Source: CAD feature listing. Evaluate the final solid. Frame: model axes, mm. Face numbers are marked on the shaded views. A direction names the side the tool comes from. Coordinates: 2 decimals unless noted, no trailing zeros. Write each loop counter-clockwise with the first axis right and the second up, starting at its lowest first coordinate (ties: lowest second). Pieces come first, ordered by that corner, then holes. Notation, with made-up numbers: M -13,-39.5 L 41,-39.5 A28 ccw 41,-15.5 Z; hole C 4.25,24.5 d5. An arc over 180 degrees is marked long. One line per item, written item: value. Start each with the question number.
Item 1: Cut plane B-B, the plane y = -25. Output: boundary loops of the cut face in (x, z).
Item 2: Cut plane A-A, the plane x = 0. Output: boundary loops of the cut face in (y, z).
Item 3: Ray query, L1, parallel to Y at x = -4.5, z = -7.75; L2, parallel to Y at x = 6.5, z = -0.6; L3, parallel to Z at x = 29.5, y = -3. Return the intervals inside material, ascending. Write a range as from..to.
Item 4: Cut plane D-D, the plane x = -19. Output: boundary loops of the cut face in (y, z), then the cut area to 3 significant figures.
Item 5: Mould query, pull axis Y, two halves, no side actions, for the marked faces 1, 2, 3 and 4. Classes: released by +Y, released by -Y, zero draft, split by the parting line, or undercut.
Item 6: Pin query (flat end, axial travel): P1, Ø6.5, axis at x = -2, z = -14, coming from the +Y side; P2, Ø5.5, axis at x = -21.5, z = -22, coming from the -Y side; P3, Ø7, axis at x = 2.5, z = -8, coming from the +Y side; P4, Ø12, axis at x = 22.5, z = -6, coming from the +Y side. Return the tip coordinate at first contact, or that it passes through.
Item 7: Set-up query: the marked faces 5, 6 and 7. Return all of +Z, -Z, +X, -X, +Y, -Y with unobstructed straight access to the full face (end or side cutting, diameter ignored); none if empty.
Item 8: Cut plane C-C, the plane z = -6.75. Output: boundary loops of the cut face in (x, y), then the cut area to 3 significant figures.
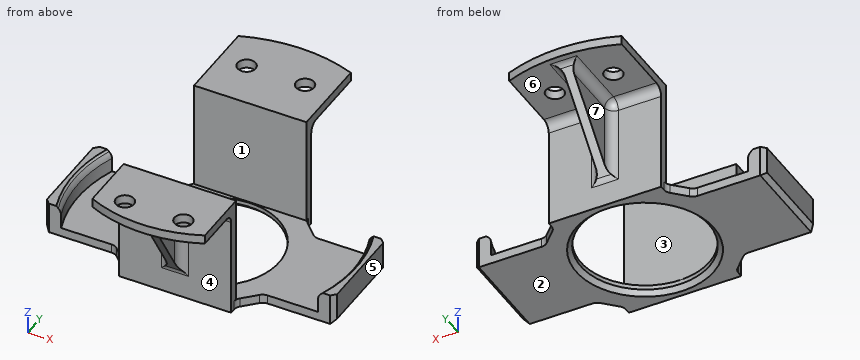
```python
from build123d import *

# Parameters (mm, degrees)
BOSS_EXTRUDE1_DEPTH     = 12.5
SKETCH2_R               = 45
SKETCH2_R_2             = 35
CUT_EXTRUDE_THIN1_DEPTH = 10
CUT_EXTRUDE1_DEPTH      = 10
BOSS_EXTRUDE2_DEPTH     = 32.275
SKETCH5_R               = 14.25
CUT_EXTRUDE2_DEPTH      = 40
CHAMFER1_SIZE           = 5
CHAMFER2_SIZE           = 1
BOSS_EXTRUDE3_DEPTH     = 5
CHAMFER3_SIZE           = 5
FILLET1_R               = 3
RIB2_REACH              = 56.318
SKETCH7_WALL_W          = 134.965083932
SKETCH7_WALL_H          = 2
RIB3_REACH              = 56.318
SKETCH8_WALL_W          = 131.736112932
SKETCH8_WALL_H          = 2
CUT_EXTRUDE3_DEPTH      = 55.318487934
CHAMFER4_SIZE           = 1
SKETCH10_R              = 2
CUT_EXTRUDE4_DEPTH      = 5
CHAMFER5_SIZE           = 1
FILLET2_R               = 2


with BuildPart() as part:
    # Sketch1 → Boss-Extrude1 (new, symmetric)
    with BuildSketch(Plane(origin=(0, 0, 0), x_dir=(0, 0, -1), z_dir=(1, 0, 0))):
        Polygon((0, 35), (0, 14.45), (24.15, 14.45), (24.15, -14.45), (0, -14.45), (0, -35), (2, -35), (2, -16.45), (26.15, -16.45), (26.15, 16.45), (2, 16.45), (2, 35), align=None)
    extrude(amount=BOSS_EXTRUDE1_DEPTH, both=True)

    # Sketch2 → Cut-Extrude-Thin1 (cut)
    with BuildSketch(Plane.XY):
        Circle(SKETCH2_R)
        Circle(SKETCH2_R_2, mode=Mode.SUBTRACT)
    extrude(amount=-CUT_EXTRUDE_THIN1_DEPTH, mode=Mode.SUBTRACT)

    # Sketch3 → Cut-Extrude1 (cut)
    with BuildSketch(Plane.XY):
        with BuildLine():
            Line((12.5, -32.691742077), (12.5, -27.271780287))
            ThreePointArc((12.5, -27.271780287), (0, -30), (-12.5, -27.271780287))
            Line((-12.5, -27.271780287), (-12.5, -32.691742077))
            ThreePointArc((-12.5, -32.691742077), (0, -35), (12.5, -32.691742077))
        make_face()
    extrude(amount=-CUT_EXTRUDE1_DEPTH, mode=Mode.SUBTRACT)

    # Sketch4 → Boss-Extrude2 (add, symmetric)
    with BuildSketch(Plane(origin=(0, 0, 0), x_dir=(0, 0, -1), z_dir=(1, 0, 0))):
        Polygon((14.075, 16.45), (14.075, 14.45), (24.15, 14.45), (24.15, -14.45), (14.075, -14.45), (14.075, -16.45), (26.15, -16.45), (26.15, 16.45), align=None)
    extrude(amount=BOSS_EXTRUDE2_DEPTH, both=True)

    # Sketch5 → Cut-Extrude2 (cut)
    with BuildSketch(Plane(origin=(0, 0, -26.15), x_dir=(-1, 0, 0), z_dir=(0, 0, -1))):
        Circle(SKETCH5_R)
    extrude(amount=-CUT_EXTRUDE2_DEPTH, mode=Mode.SUBTRACT)

    # Chamfer1
    chamfer1_edges = [part.edges().sort_by_distance(p)[0] for p in [
        (12.5, -15.45, -14.075),
        (-12.5, -15.45, -14.075),
        (12.5, 15.45, -14.075),
        (-12.5, 15.45, -14.075),
    ]]
    chamfer(chamfer1_edges, length=CHAMFER1_SIZE)

    # Chamfer2
    chamfer2_edges = [part.edges().sort_by_distance(p)[0] for p in [
        (14.25, 0, -26.15),
    ]]
    chamfer(chamfer2_edges, length=CHAMFER2_SIZE)

    # Sketch6 → Boss-Extrude3 (add)
    with BuildSketch(Plane.XY.offset(-24.15)):
        with BuildLine():
            Line((-32.275, -14.45), (-32.275, 14.45))
            Line((-32.275, 14.45), (-26.774579829, 14.45))
            ThreePointArc((-26.774579829, 14.45), (-30.425, 0), (-26.774579829, -14.45))
            Line((-26.774579829, -14.45), (-32.275, -14.45))
        make_face()
        with BuildLine():
            Line((32.275, -14.45), (26.774579829, -14.45))
            ThreePointArc((26.774579829, -14.45), (30.425, 0), (26.774579829, 14.45))
            Line((26.774579829, 14.45), (32.275, 14.45))
            Line((32.275, 14.45), (32.275, -14.45))
        make_face()
    extrude(amount=BOSS_EXTRUDE3_DEPTH)

    # Chamfer3
    chamfer3_edges = [part.edges().sort_by_distance(p)[0] for p in [
        (-32.275, 16.45, -20.1125),
        (-32.275, -16.45, -20.1125),
        (32.275, -16.45, -20.1125),
        (32.275, 16.45, -20.1125),
    ]]
    chamfer(chamfer3_edges, length=CHAMFER3_SIZE)

    # Fillet1
    fillet1_edges = [part.edges().sort_by_distance(p)[0] for p in [
        (-28.024789914, -14.45, -19.15),
        (28.024789914, -14.45, -19.15),
        (28.024789914, 14.45, -19.15),
        (-28.024789914, 14.45, -19.15),
    ]]
    fillet(fillet1_edges, radius=FILLET1_R)

    # Sketch7 wall → Rib2 (add, up to next)
    with BuildSketch(Plane(origin=(0, 24.570871039, -11.05625), x_dir=(0, -0.667612213603, -0.744509188827), z_dir=(0, 0.744509188827, -0.667612213603)), mode=Mode.PRIVATE) as rib2_sk1:
        Rectangle(SKETCH7_WALL_W, SKETCH7_WALL_H)
    rib2_tool1 = extrude(rib2_sk1.sketch, amount=-RIB2_REACH, mode=Mode.PRIVATE) - part.part
    add(rib2_tool1.solids().sort_by_distance((0, 24.570871039, -11.05625))[0])

    # Sketch8 wall → Rib3 (add, up to next)
    with BuildSketch(Plane(origin=(0, -21.860890144, -11.05625), x_dir=(0, -0.512901558692, 0.858447430593), z_dir=(0, -0.858447430593, -0.512901558692)), mode=Mode.PRIVATE) as rib3_sk1:
        Rectangle(SKETCH8_WALL_W, SKETCH8_WALL_H)
    rib3_tool1 = extrude(rib3_sk1.sketch, amount=-RIB3_REACH, mode=Mode.PRIVATE) - part.part
    add(rib3_tool1.solids().sort_by_distance((0, -21.860890144, -11.05625))[0])

    # Sketch9 → Cut-Extrude3 (cut, through all)
    with BuildSketch(Plane(origin=(0, 0, -26.15), x_dir=(-1, 0, 0), z_dir=(0, 0, -1))):
        Polygon((12.5, 14.45), (12.5, 16.45), (27.275, 16.45), (32.275, 11.45), (32.275, 10.45), (16.5, 10.45), align=None)
        Polygon((-27.275, 16.45), (-32.275, 11.45), (-32.275, 10.45), (-16.5, 10.45), (-12.5, 14.45), (-12.5, 16.45), align=None)
        Polygon((27.275, -16.45), (32.275, -11.45), (32.275, -10.45), (16.5, -10.45), (12.5, -14.45), (12.5, -16.45), align=None)
        Polygon((-12.5, -14.45), (-12.5, -16.45), (-27.275, -16.45), (-32.275, -11.45), (-32.275, -10.45), (-16.5, -10.45), align=None)
    extrude(amount=-CUT_EXTRUDE3_DEPTH, mode=Mode.SUBTRACT)

    # Chamfer4
    chamfer4_edges = [part.edges().sort_by_distance(p)[0] for p in [
        (30.425, 0, -19.15),
        (-30.425, 0, -19.15),
    ]]
    chamfer(chamfer4_edges, length=CHAMFER4_SIZE)

    # Sketch10 → Cut-Extrude4 (cut)
    with BuildSketch(Plane(origin=(0, 0, -2), x_dir=(-1, 0, 0), z_dir=(0, 0, -1))):
        with Locations((6.5, 25)):
            Circle(SKETCH10_R)
        with Locations((-6.5, 25)):
            Circle(SKETCH10_R)
        with Locations((-6.5, -25)):
            Circle(SKETCH10_R)
        with Locations((6.5, -25)):
            Circle(SKETCH10_R)
    extrude(amount=-CUT_EXTRUDE4_DEPTH, mode=Mode.SUBTRACT)

    # Chamfer5
    chamfer5_edges = [part.edges().sort_by_distance(p)[0] for p in [
        (-32.275, 10.45, -22.65),
        (32.275, 10.45, -22.65),
        (-32.275, 0, -26.15),
        (-32.275, -10.45, -22.65),
        (32.275, 0, -26.15),
        (32.275, -10.45, -22.65),
    ]]
    chamfer(chamfer5_edges, length=CHAMFER5_SIZE)

    # Fillet2
    fillet2_edges = [part.edges().sort_by_distance(p)[0] for p in [
        (-30.425, 0, -20.15),
        (30.425, 0, -20.15),
        (12.5, 14.45, -25.15),
        (-12.5, 14.45, -25.15),
        (-12.5, -14.45, -25.15),
        (12.5, -14.45, -25.15),
        (16.5, -10.45, -25.15),
        (16.5, 10.45, -25.15),
        (-16.5, 10.45, -25.15),
        (-16.5, -10.45, -25.15),
        (6.75, -16.45, -2),
        (-6.75, -16.45, -2),
        (-6.75, 16.45, -2),
        (6.75, 16.45, -2),
        (0, -27.271780287, -2),
        (0, 32.691742077, -2),
        (0, 16.45, -20.112500001),
        (0, -16.45, -20.112500001),
        (1, -21.860890144, -2),
        (1, -16.45, -11.05625),
        (-1, -21.860890144, -2),
        (-1, -16.45, -11.05625),
        (-1, 24.570871039, -2),
        (-1, 16.45, -11.05625),
        (1, 24.570871039, -2),
        (1, 16.45, -11.05625),
    ]]
    fillet(fillet2_edges, radius=FILLET2_R)


solid = part.part
```
From the geometry:
1. outline: M -12.5,-2 L -8.5,-2 L -8.5,0 L -12.5,0 Z; M -4.5,-2 L -3,-2 A2 cw -1,-4 L -1,-5.8 L 1,-5.8 L 1,-4 A2 cw 3,-2 L 4.5,-2 L 4.5,0 L -4.5,0 Z; M 8.5,-2 L 12.5,-2 L 12.5,0 L 8.5,0 Z
2. outline: M -30,-2 L -28.41,-2 A2 cw -26.69,-2.97 L -16.73,-19.64 A2 cw -16.45,-20.66 L -16.45,-26.15 L -15.25,-26.15 L -14.25,-25.15 L -14.25,-24.15 L -14.45,-24.15 L -14.45,0 L -30,0 Z; M 14.25,-25.15 L 15.25,-26.15 L 16.45,-26.15 L 16.45,-20.88 A2 cw 16.96,-19.54 L 32.1,-2.66 A2 cw 33.58,-2 L 35,-2 L 35,0 L 14.45,0 L 14.45,-24.15 L 14.25,-24.15 Z
3. L1: y = -16.45..-14.45, 14.45..16.45
3. L2: y = -29.29..-27, -23..-14.45, 14.45..23, 27..34.39
3. L3: z = -26.15..-24.15
4. outline: M -10.45,-26.15 L 10.45,-26.15 L 10.45,-24.15 L -10.45,-24.15 Z
4. area: 41.8 mm²
5. face 1: undercut
5. face 2: zero draft
5. face 3: undercut
5. face 4: released by -Y
6. P1: stops at y = 24.7
6. P2: stops at y = -10.45
6. P3: stops at y = 30.15
6. P4: passes through
7. face 5: +Z, -Z, +X, +Y, -Y
7. face 6: -Z, +Y
7. face 7: -Z, -X, +Y
8. outline: M -12.5,-16.45 L -3,-16.45 A2 cw -1,-18.45 L -1,-24.43 L 1,-24.43 L 1,-18.45 A2 cw 3,-16.45 L 12.5,-16.45 L 12.5,-14.45 L -12.5,-14.45 Z; M -12.5,14.45 L 12.5,14.45 L 12.5,16.45 L 3,16.45 A2 cw 1,18.45 L 1,28.43 L -1,28.43 L -1,18.45 A2 cw -3,16.45 L -12.5,16.45 Z
8. area: 143 mm²
